```python
from build123d import *

# Parameters (mm, degrees)
SKETCH2_R           = 39.487475
BOSS_EXTRUDE1_DEPTH = 5.842
FILLET1_R           = 0.79375
SKETCH4_W           = 5.742
SKETCH4_H           = 12.5
CUT_EXTRUDE3_DEPTH  = 163.986308211
SKETCH5_R           = 0.1984375
CUT_EXTRUDE4_DEPTH  = 163.986308211


with BuildPart() as part:
    # Sketch2 → Boss-Extrude1 (new body)
    with BuildSketch(Plane(origin=(0, 0, 0), x_dir=(0, 0, -1), z_dir=(1, 0, 0))):
        with BuildLine():
            Line((81.02619141, 88.258519733), (35.921024484, 114.3))
            ThreePointArc((35.921024484, 114.3), (0, 63.5), (-35.921024484, 114.3))
            Line((-35.921024484, 114.3), (-81.02619141, 88.258519733))
            ThreePointArc((-81.02619141, 88.258519733), (-54.99261314, 31.75), (-116.947215895, 26.041480267))
            Line((-116.947215895, 26.041480267), (-116.947215895, -26.041480267))
            ThreePointArc((-116.947215895, -26.041480267), (-54.99261314, -31.75), (-81.02619141, -88.258519733))
            Line((-81.02619141, -88.258519733), (-35.921024484, -114.3))
            ThreePointArc((-35.921024484, -114.3), (0, -63.5), (35.921024484, -114.3))
            Line((35.921024484, -114.3), (81.02619141, -88.258519733))
            ThreePointArc((81.02619141, -88.258519733), (54.99261314, -31.75), (116.947215895, -26.041480267))
            Line((116.947215895, -26.041480267), (116.947215895, 26.041480267))
            ThreePointArc((116.947215895, 26.041480267), (54.99261314, 31.75), (81.02619141, 88.258519733))
        make_face()
        Circle(SKETCH2_R, mode=Mode.SUBTRACT)
    extrude(amount=BOSS_EXTRUDE1_DEPTH)

    # Fillet1
    fillet1_edges = [part.edges().sort_by_distance(p)[0] for p in [
        (2.921, 88.258519733, 81.02619141),
        (2.921, 114.3, 35.921024484),
        (2.921, 114.3, -35.921024484),
        (2.921, 88.258519733, -81.02619141),
        (2.921, 26.041480267, -116.947215895),
        (2.921, -26.041480267, -116.947215895),
        (2.921, -88.258519733, -81.02619141),
        (2.921, -114.3, -35.921024484),
        (2.921, -114.3, 35.921024484),
        (2.921, -88.258519733, 81.02619141),
        (2.921, -26.041480267, 116.947215895),
        (2.921, 26.041480267, 116.947215895),
    ]]
    fillet(fillet1_edges, radius=FILLET1_R)

    # Sketch4 → Cut-Extrude3 (cut, through all)
    with BuildSketch(Plane(origin=(5.842, 0, 0), x_dir=(0, 0, -1), z_dir=(1, 0, 0))):
        Polygon((47.971249286, -31.011358934), (50.842249286, -26.038641066), (40.016931739, -19.788641066), (37.145931739, -24.761358934), align=None)
        with Locations((0, 50.8)):
            Rectangle(SKETCH4_W, SKETCH4_H)
        Polygon((-50.842249286, -26.038641066), (-47.971249286, -31.011358934), (-37.145931739, -24.761358934), (-40.016931739, -19.788641066), align=None)
    extrude(amount=-CUT_EXTRUDE3_DEPTH, mode=Mode.SUBTRACT)

    # Sketch5 → Cut-Extrude4 (cut, through all)
    with BuildSketch(Plane(origin=(5.842, 0, 0), x_dir=(0, 0, -1), z_dir=(1, 0, 0))):
        with Locations((2.871, 57.05)):
            Circle(SKETCH5_R)
        with Locations((-2.871, 57.05)):
            Circle(SKETCH5_R)
        with Locations((-2.871, 44.55)):
            Circle(SKETCH5_R)
        with Locations((2.871, 44.55)):
            Circle(SKETCH5_R)
        with Locations((47.971249286, -31.011358934)):
            Circle(SKETCH5_R)
        with Locations((50.842249286, -26.038641066)):
            Circle(SKETCH5_R)
        with Locations((40.016931739, -19.788641066)):
            Circle(SKETCH5_R)
        with Locations((37.145931739, -24.761358934)):
            Circle(SKETCH5_R)
        with Locations((-50.842249286, -26.038641066)):
            Circle(SKETCH5_R)
        with Locations((-47.971249286, -31.011358934)):
            Circle(SKETCH5_R)
        with Locations((-37.145931739, -24.761358934)):
            Circle(SKETCH5_R)
        with Locations((-40.016931739, -19.788641066)):
            Circle(SKETCH5_R)
    extrude(amount=-CUT_EXTRUDE4_DEPTH, mode=Mode.SUBTRACT)


solid = part.part
```
Here's how the part is built. I have some questions about the finished solid (model axes, mm). A direction names the side the tool comes from. Coordinates: 2 decimals unless noted, no trailing zeros. Loops run counter-clockwise (first coordinate to the right, second up) from the corner with the lowest first, then second, coordinate; pieces in that order, holes last. Notation, with made-up numbers: (19, 41.5) -> (62, 41.5) arc R14 cw to (62, 54.5) -> close; hole circle Ø7 at (68.25, 0.25). An arc over 180 degrees is marked (long way). Return JSON: item names as keys, results as strings.
1) If we section it at C-C, the plane y = -50.8: Write out the boundary of the cut face in (x, z).
Results below:
{"outline": "(0, -49.89) -> (5.84, -49.89) -> (5.84, 49.89) -> (0, 49.89) -> close"}
2) If we section it at A-A, the plane y = 0: Write out the boundary of the cut face in (x, z), then the cut area to 3 significant figures.
Results below:
{"outline": "(0, -116.95) -> (5.84, -116.95) -> (5.84, -39.49) -> (0, -39.49) -> close; (0, 39.49) -> (5.84, 39.49) -> (5.84, 116.95) -> (0, 116.95) -> close", "area": "905 mm²"}
3) Thinking about a two-plate mould opening in Z: for faces 3 (the face through (3, 0, -116.947)), 4 (the face through (2.88, 63.513, -0.99)), 5 (the face through (5.842, 43, 1)), 6 (the face through (2.88, -101.111, 58.764)), which applies, +Z half, -Z half, draft (parallel to the pull), parting line (faces both ways), or undercut?
Results below:
{"face 3": "-Z half", "face 4": "undercut", "face 5": "draft", "face 6": "+Z half"}
4) If we section it at D-D, the plane y = 94: Write out the boundary of the cut face in (x, z), then the cut area to 3 significant figures.
Results below:
{"outline": "(0, -71.08) -> (5.84, -71.08) -> (5.84, -37.33) -> (0, -37.33) -> close; (0, 37.33) -> (5.84, 37.33) -> (5.84, 71.08) -> (0, 71.08) -> close", "area": "394 mm²"}
5) If we section it at B-B, the plane z = 0: Write out the boundary of the cut face in (x, y).
Results below:
{"outline": "(0, -63.5) -> (5.84, -63.5) -> (5.84, -39.49) -> (0, -39.49) -> close; (0, 39.49) -> (5.84, 39.49) -> (5.84, 44.55) -> (0, 44.55) -> close; (0, 57.05) -> (5.84, 57.05) -> (5.84, 63.5) -> (0, 63.5) -> close"}
6) I need wall thicknesses on line 1 (Y direction, x = 4.15, z = 77); line 2 (Z direction, x = 2.7, y = 50); line 3 (Z direction, x = 0.9, y = 0.5). Which ranges of each line are inside material? Lowest first, please. Write a range as from..to.
Results below:
{"line 1": "-90.58..-87.28, -14.32..14.32, 87.28..90.58", "line 2": "-49.9..-2.87, 2.87..49.9", "line 3": "-116.95..-39.48, 39.48..116.95"}
7) Will these pins go through, and if not, where does the flat tip stop? pin 1 (1 mm diameter, centred on x = 1, z = 29, fed in from -Y); pin 2 (2.5 mm diameter, centred on x = 4, z = 0.5, fed in from +Y); pin 3 (3 mm diameter, centred on x = 2.5, y = 38, fed in from -Z).
Results below:
{"pin 1": "y = -77.49", "pin 2": "y = 63.54", "pin 3": "z = -52.67"}
8) For faces 1 (the face through (0, 43, 1)), 2 (the face through (3, 57.05, 0)), which set-ups out of +Z, -Z, +X, -X, +Y, -Y let a thin tool reach every point of the face, with its end or its side?
Results below:
{"face 1": "+Z, -Z, -X, +Y, -Y", "face 2": "+X, -X"}
